from build123d import *
from build123d.topology import SkipClean

# Parameters (mm, degrees)
SKETCH1_R           = 5.5
BOSS_EXTRUDE1_DEPTH = 0.25
SKETCH2_R           = 1.5
BOSS_EXTRUDE2_DEPTH = 2.5
SKETCH3_R           = 0.75
CUT_EXTRUDE1_DEPTH  = 9.336666
BOSS_EXTRUDE3_START = 6.5
BOSS_EXTRUDE3_DEPTH = 6.5
CIRPATTERN1_COUNT   = 6
BOSS_EXTRUDE6_START = 0.25
SKETCH5_R           = 5.5
SKETCH5_R_2         = 4
BOSS_EXTRUDE6_DEPTH = 0.25


with BuildPart() as part:
    # Sketch1 → Boss-Extrude1 (new, symmetric)
    with BuildSketch(Plane(origin=(0, 0, 0), x_dir=(0, 0, -1), z_dir=(1, 0, 0))):
        Circle(SKETCH1_R)
    extrude(amount=BOSS_EXTRUDE1_DEPTH, both=True)

    # Sketch2 → Boss-Extrude2 (add)
    with BuildSketch(Plane.ZY.offset(0.25)):
        Circle(SKETCH2_R)
    extrude(amount=BOSS_EXTRUDE2_DEPTH)

    # Sketch3 → Cut-Extrude1 (cut, through all)
    with BuildSketch(Plane.ZY.offset(2.75)):
        Circle(SKETCH3_R)
    extrude(amount=-CUT_EXTRUDE1_DEPTH, mode=Mode.SUBTRACT)

    # Sketch4 → Boss-Extrude3 (add)
    with BuildSketch(Plane(origin=(0.25, 0, 0), x_dir=(0, 0, -1), z_dir=(1, 0, 0)).offset(BOSS_EXTRUDE3_START)):
        with BuildLine():
            Line((-5.5, 0), (-3.02, 0))
            Line((-3.02, 0), (-3.02, 0.15))
            Line((-3.02, 0.15), (-5.347896783, 0.15))
            ThreePointArc((-5.347896783, 0.15), (-5.196916014, 1.270654927), (-4.813771652, 2.334545455))
            Line((-4.813771652, 2.334545455), (-4.948737213, 2.4))
            ThreePointArc((-4.948737213, 2.4), (-5.360412982, 1.231248417), (-5.5, 0))
        make_face()
    boss_extrude3 = extrude(amount=-BOSS_EXTRUDE3_DEPTH)

    # CirPattern1: Boss-Extrude3 ×6 about axis
    with SkipClean():  # the faces are left unmerged after this step: merging them gives an invalid solid
        cirpattern1_axis = Axis((0, 0, 0), (1, 0, 0))
        for i in range(1, CIRPATTERN1_COUNT):
            add(boss_extrude3.rotate(cirpattern1_axis, i * 360 / CIRPATTERN1_COUNT))

    # Sketch5 → Boss-Extrude6 (add)
    with SkipClean():  # the faces are left unmerged after this step: merging them gives an invalid solid
        with BuildSketch(Plane(origin=(6.75, 0, 0), x_dir=(0, 0, -1), z_dir=(1, 0, 0)).offset(BOSS_EXTRUDE6_START)):
            Circle(SKETCH5_R)
            Circle(SKETCH5_R_2, mode=Mode.SUBTRACT)
        extrude(amount=-BOSS_EXTRUDE6_DEPTH)


solid = part.part
Input: part model. Units: mm. Frame: model coordinates. A direction names the side the tool comes from. Give positions to 0.01 mm unless a question says otherwise; leave off trailing zeros. Write each loop counter-clockwise with the first axis right and the second up, starting at its lowest first coordinate (ties: lowest second). Pieces come first, ordered by that corner, then holes. Notation, with made-up numbers: M 28.5,-29 L 47.5,-29 A16 ccw 47.5,-4 Z; hole C 60.5,12 d8. An arc over 180 degrees is marked long. Use one line per item in the form item = value.
1. First-contact query: P1, Ø1.5, axis at x = 5, z = -1, coming from the -Y side; P2, Ø0.6, axis at y = 5, z = -1, coming from the -X side; P3, Ø0.5, axis at y = 3, z = 1.5, coming from the +X side. Flat tips, straight axial feed; report the tip coordinate or a pass-through.
Outcome:
P1 = -5.49
P2 = -0.25
P3 = 6.75
2. Cut plane A-A on z = 0. Return loops of the section in (x, y).
Outcome:
outline = M -2.75,-1.5 L -0.25,-1.5 L -0.25,-5.5 L 0.25,-5.5 L 0.25,-0.75 L -2.75,-0.75 Z; M -2.75,0.75 L 0.25,0.75 L 0.25,5.5 L -0.25,5.5 L -0.25,1.5 L -2.75,1.5 Z; M 6.75,-5.5 L 7,-5.5 L 7,-4 L 6.75,-4 Z; M 6.75,4 L 7,4 L 7,5.5 L 6.75,5.5 Z
3. Cut plane B-B on z = 3.25. Return loops of the section in (x, y), and give its area (3 significant figures).
Outcome:
outline = M -0.25,-4.44 L 7,-4.44 L 7,-2.33 L 6.75,-2.33 L 6.75,-4.25 L 0.25,-4.25 L 0.25,0 L 6.75,0 L 6.75,0.15 L 0.25,0.15 L 0.25,4.44 L -0.25,4.44 Z; M 6.75,2.33 L 7,2.33 L 7,4.44 L 6.75,4.44 Z
area = 7.68 mm²
4. Cut plane C-C on x = 4. State how many separate pieces and enclosed holes the cut face has, and give its area (3 significant figures).
Outcome:
separate_pieces = 6
enclosed_holes = 0
area = 4.30 mm²
5. Ray query, L1, parallel to X at y = 4.25, z = -2; L2, parallel to Y at x = 6.95, z = 0. Return the intervals inside material, ascending.
Outcome:
L1 = -0.25 to 0.25, 6.75 to 7
L2 = -5.5 to -4, 4 to 5.5
6. Reachability of faces 4 (the face through (-0.25, -1.1, 1.3)), 5 (the face through (3.546, -3.534, 2.214)), 6 (the face through (3.546, 1.498, 5.136)) from +Z, -Z, +X, -X, +Y, -Y: full face, straight path, thin tool, end or side. Return the list, or none.
Outcome:
face_4 = -X
face_5 = none
face_6 = -Z
7. Mould query, pull axis X, two halves, no side actions, for faces 1 (the face through (7, -2, 4)), 2 (the face through (-1.27, 0.03, -0.75)), 3 (the face through (3.546, 3.704, 2.139)). Classes: released by +X, released by -X, zero draft, split by the parting line, or undercut.
Outcome:
face_1 = released by +X
face_2 = zero draft
face_3 = undercut
8. Cut plane D-D on x = -1.25. Return loops of the section in (y, z), and give its area (3 significant figures).
Outcome:
outline = C 0,0 d3; hole C 0,0 d1.5
area = 5.30 mm²
